Geometry: final body of the model. Coordinates: model frame, mm. Round coordinates to 2 decimals unless told otherwise and drop trailing zeros. Write each loop counter-clockwise with the first axis right and the second up, starting at its lowest first coordinate (ties: lowest second). Pieces come first, ordered by that corner, then holes. Notation, with made-up numbers: (-39, 16.25) -> (12, 16.25) arc R25 ccw to (12, 38.25) -> close; hole circle Ø3 at (-19.75, -35.5). An arc over 180 degrees is marked (long way). Use one line per item in the form item = value. Start each with the question number.
1. Line query: L1, parallel to Z at x = -60, y = 71. Output: solid intervals per line, ascending.
2. Pin query (flat end, axial travel): pin 1 Ø3 at (x, y) = (7.5, 24) entering from +Z. Return the tip coordinate at first contact, or that it passes through.
3. Cut plane A-A, the plane y = -21.5. Return the cut outline in (x, z), plus the area to 3 significant figures.
```python
from build123d import *

# Parameters (mm, degrees)
F0_W     = 203.2
F0_H     = 203.2
F1_DEPTH = 6.35
F2_R     = 6.35
F3_DEPTH = 3.81


with BuildPart() as f1:
    # F0 (on Top) → F1 (new body)
    with BuildSketch(Plane.XY):
        Rectangle(F0_W, F0_H)
    extrude(amount=F1_DEPTH)

    # F2 (on face) → F3 (join)
    with BuildSketch(Plane.XY.offset(6.35)):
        with Locations((-88.9, 88.9)):
            Circle(F2_R)
        with Locations((-88.696807, 63.500813)):
            Circle(F2_R)
        with Locations((-88.493613, 38.101626)):
            Circle(F2_R)
        with Locations((-88.29042, 12.702438)):
            Circle(F2_R)
        with Locations((-88.087226, -12.696749)):
            Circle(F2_R)
        with Locations((-87.884033, -38.095936)):
            Circle(F2_R)
        with Locations((-87.680839, -63.495123)):
            Circle(F2_R)
        with Locations((-87.477646, -88.894311)):
            Circle(F2_R)
        with Locations((-63.5, 88.9)):
            Circle(F2_R)
        with Locations((-63.296807, 63.500813)):
            Circle(F2_R)
        with Locations((-63.093613, 38.101626)):
            Circle(F2_R)
        with Locations((-62.89042, 12.702438)):
            Circle(F2_R)
        with Locations((-62.687226, -12.696749)):
            Circle(F2_R)
        with Locations((-62.484033, -38.095936)):
            Circle(F2_R)
        with Locations((-62.280839, -63.495123)):
            Circle(F2_R)
        with Locations((-62.077646, -88.894311)):
            Circle(F2_R)
        with Locations((-38.1, 88.9)):
            Circle(F2_R)
        with Locations((-37.896807, 63.500813)):
            Circle(F2_R)
        with Locations((-37.693613, 38.101626)):
            Circle(F2_R)
        with Locations((-37.49042, 12.702438)):
            Circle(F2_R)
        with Locations((-37.287226, -12.696749)):
            Circle(F2_R)
        with Locations((-37.084033, -38.095936)):
            Circle(F2_R)
        with Locations((-36.880839, -63.495123)):
            Circle(F2_R)
        with Locations((-36.677646, -88.894311)):
            Circle(F2_R)
        with Locations((-12.7, 88.9)):
            Circle(F2_R)
        with Locations((-12.496807, 63.500813)):
            Circle(F2_R)
        with Locations((-12.293613, 38.101626)):
            Circle(F2_R)
        with Locations((-12.09042, 12.702438)):
            Circle(F2_R)
        with Locations((-11.887226, -12.696749)):
            Circle(F2_R)
        with Locations((-11.684033, -38.095936)):
            Circle(F2_R)
        with Locations((-11.480839, -63.495123)):
            Circle(F2_R)
        with Locations((-11.277646, -88.894311)):
            Circle(F2_R)
        with Locations((12.7, 88.9)):
            Circle(F2_R)
        with Locations((12.903193, 63.500813)):
            Circle(F2_R)
        with Locations((13.106387, 38.101626)):
            Circle(F2_R)
        with Locations((13.30958, 12.702438)):
            Circle(F2_R)
        with Locations((13.512774, -12.696749)):
            Circle(F2_R)
        with Locations((13.715967, -38.095936)):
            Circle(F2_R)
        with Locations((13.919161, -63.495123)):
            Circle(F2_R)
        with Locations((14.122354, -88.894311)):
            Circle(F2_R)
        with Locations((38.1, 88.9)):
            Circle(F2_R)
        with Locations((38.303193, 63.500813)):
            Circle(F2_R)
        with Locations((38.506387, 38.101626)):
            Circle(F2_R)
        with Locations((38.70958, 12.702438)):
            Circle(F2_R)
        with Locations((38.912774, -12.696749)):
            Circle(F2_R)
        with Locations((39.115967, -38.095936)):
            Circle(F2_R)
        with Locations((39.319161, -63.495123)):
            Circle(F2_R)
        with Locations((39.522354, -88.894311)):
            Circle(F2_R)
        with Locations((63.5, 88.9)):
            Circle(F2_R)
        with Locations((63.703193, 63.500813)):
            Circle(F2_R)
        with Locations((63.906387, 38.101626)):
            Circle(F2_R)
        with Locations((64.10958, 12.702438)):
            Circle(F2_R)
        with Locations((64.312774, -12.696749)):
            Circle(F2_R)
        with Locations((64.515967, -38.095936)):
            Circle(F2_R)
        with Locations((64.719161, -63.495123)):
            Circle(F2_R)
        with Locations((64.922354, -88.894311)):
            Circle(F2_R)
        with Locations((88.9, 88.9)):
            Circle(F2_R)
        with Locations((89.103193, 63.500813)):
            Circle(F2_R)
        with Locations((89.306387, 38.101626)):
            Circle(F2_R)
        with Locations((89.50958, 12.702438)):
            Circle(F2_R)
        with Locations((89.712774, -12.696749)):
            Circle(F2_R)
        with Locations((89.915967, -38.095936)):
            Circle(F2_R)
        with Locations((90.119161, -63.495123)):
            Circle(F2_R)
        with Locations((90.322354, -88.894311)):
            Circle(F2_R)
    extrude(amount=F3_DEPTH)


solid = f1.part
```
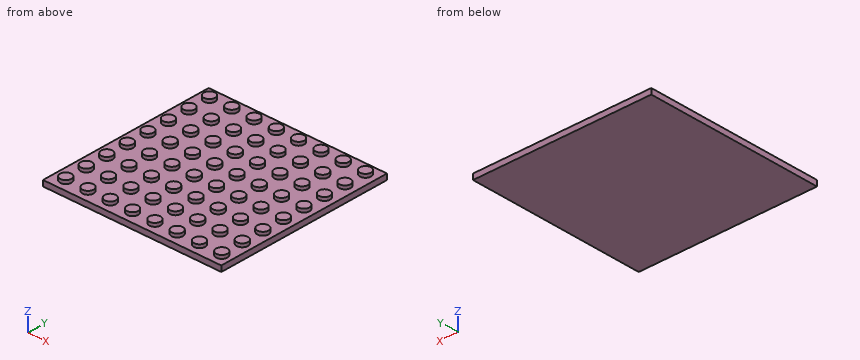
Outcome:
q1.L1 = 0 to 6.35
q2.pin_1 = 6.35
q3.outline = (-101.6, 0) -> (101.6, 0) -> (101.6, 6.35) -> (-101.6, 6.35) -> close
q3.area = 1,290 mm^2
